Check sheet for the modelled part. Datum: model origin and axes. Units: mm. Give positions to 0.01 mm unless a question says otherwise; leave off trailing zeros. Write each loop counter-clockwise with the first axis right and the second up, starting at its lowest first coordinate (ties: lowest second). Pieces come first, ordered by that corner, then holes. Notation, with made-up numbers: M -3,49 L 29,49 A10 ccw 29,63 Z; hole C 56.5,11 d5. An arc over 180 degrees is marked long. Use CSV: the item, a comma, the result in double quotes. Start each with the question number.
1. Cross-section at A-A, the plane x = -143. Enter the section's corners in (y, z).
2. Depth check by flat-ended pin: P1, Ø11, axis at x = -143, y = 34.44, coming from the +Z side. Enter the tip coordinate at first touch or a pass-through.
3. Scan lines: line 1 (Y direction, x = -143, z = -3.75); line 2 (Y direction, x = -147.5, z = -3.65). Record each from-to range of solid material in increasing order.
4. Mould release check, pull along X, two halves, no side actions. Record for faces 1 (the face through (-138.239, -10.567, -2.465)), 2 (the face through (-2, 4, 0)): +X half, -X half, draft (parallel to the pull), parting line (faces both ways), or undercut.
from build123d import *

# Parameters (mm, degrees)
SKETCH1_W          = 325
SKETCH1_H          = 550
SKETCH1_R          = 6
BASE_FLANGE1_DEPTH = 5


# Sheet-metal steps are written as plain solids
with BuildPart() as part:
    # Sketch1 → Base-Flange1 (new body)
    with BuildSketch(Plane.XY):
        Rectangle(SKETCH1_W, SKETCH1_H)
        with Locations(Location((-143, -14.218036313, 0), (0, 0, 180))):
            Circle(SKETCH1_R, mode=Mode.SUBTRACT)
        with Locations(Location((-143, 34.435225531, 0), (0, 0, 180))):
            Circle(SKETCH1_R, mode=Mode.SUBTRACT)
    extrude(amount=-BASE_FLANGE1_DEPTH)


solid = part.part
Worked answers:
1,outline,"M -275,-5 L -20.22,-5 L -20.22,0 L -275,0 Z; M -8.22,-5 L 28.44,-5 L 28.44,0 L -8.22,0 Z; M 40.44,-5 L 275,-5 L 275,0 L 40.44,0 Z"
2,P1,"passes through"
3,line 1,"y = -275 to -20.22, -8.22 to 28.44, 40.44 to 275"
3,line 2,"y = -275 to -18.19, -10.25 to 30.47, 38.4 to 275"
4,face 1,"undercut"
4,face 2,"draft"
